Read the model definition and answer for the solid it produces. Units are mm, in the model's axes. Face numbers are marked on the shaded views. A direction names the side the tool comes from. Coordinates: 2 decimals unless noted, no trailing zeros. Loops run counter-clockwise (first coordinate to the right, second up) from the corner with the lowest first, then second, coordinate; pieces in that order, holes last.
Q1. Which of the six approach directions +Z, -Z, +X, -X, +Y, -Y give full straight-line access (tool end or side, diameter ignored) to the marked faces 1 and 2?
Q2. Section C-C (y = 3.5) is taken. Give the vertices of the cut face in (x, z), then the cut area to 3 significant figures.
Q3. Section A-A (z = 0) is taken. Give the vertices of the cut face in (x, y).
Q4. Section B-B (x = 0) is taken. Give the vertices of the cut face in (y, z).
Q5. Straight lines are drawn through the part: line 1 (Y direction, x = -0.75, z = -1.35); line 2 (Y direction, x = -1.2, z = -0.05); line 3 (X direction, y = 2, z = 0.1). For each, find the intervals that lie inside material, in ascending order.
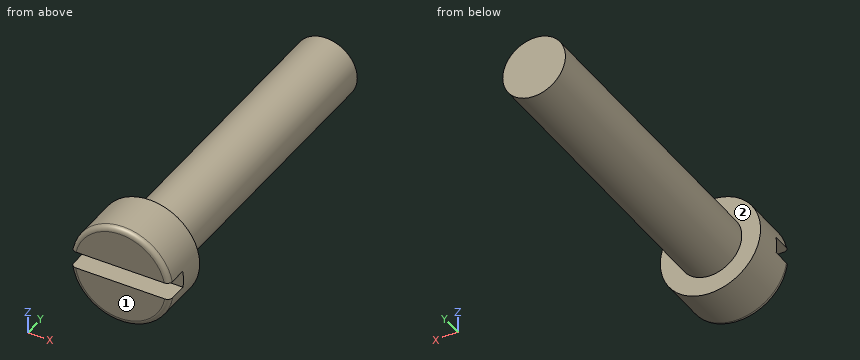
Solid Edge part; units mm, degrees
sketch "Sketch1" plane through (0, 0, 0) normal (0, -1, 0) x (1, 0, 0)
  circle A0 centre (0, 0) radius 2
extrude "Protrusion1" add sketch "Sketch1" along normal blind 2
sketch "Sketch2" plane through (0, 0, 0) normal (0, -1, 0) x (1, 0, 0)
  circle A0 centre (0, 0) radius 1.25
extrude "ExtrudedProtrusion_2" add sketch "Sketch2" against normal blind 12
sketch "Sketch3" plane through (0, -2, 0) normal (0, -1, 0) x (1, 0, 0)
  line L0 (-1.9642, 0.3767) -> (1.9642, 0.3767)
  line L1 (1.9772, -0.3013) -> (-1.9772, -0.3013)
  arc A0 (1.9642, 0.3767) -> (1.9772, -0.3013) centre (0, 0) cw
extrude "ExtrudedCutout_1" cut sketch "Sketch3" against normal blind 0.9 material side at (0, -2, 0.3267)
cosmetic_thread "Thread1"
fillet "Round_1" radius 0.2 2 edges at (0, -2, 2) (0, -2, -2)
properties material "Nylon, general purpose"
Numbers:
1. face 1: +Z, -Z, +X, -X, -Y
1. face 2: +Y
2. outline: circle Ø2.5 at (0, 0)
2. area: 4.91 mm2
3. outline: (-2, -1.1) - (2, -1.1) - (2, 0) - (1.25, 0) - (1.25, 12) - (-1.25, 12) - (-1.25, 0) - (-2, 0) - close
4. outline: (-2, -1.8) arc R0.2 ccw to (-1.8, -2) - (0, -2) - (0, -1.25) - (12, -1.25) - (12, 1.25) - (0, 1.25) - (0, 2) - (-1.8, 2) arc R0.2 ccw to (-2, 1.8) - (-2, 0.38) - (-1.1, 0.38) - (-1.1, -0.3) - (-2, -0.3) - close
5. line 1: y = -2 to 0
5. line 2: y = -1.1 to 12
5. line 3: x = -1.25 to 1.25
